from build123d import *

# Parameters (mm, degrees)
F0_R           = 12.7
F1_DEPTH       = 101.6
F3_R           = 10.16
F4_D           = 6.35
F4_START       = 2.7819668
F4_CSINK_D     = 19.05
F4_CSINK_ANGLE = 44.9


with BuildPart() as f1:
    # F0 (on Top) → F1 (new body)
    with BuildSketch(Plane.XY):
        Circle(F0_R)
    extrude(amount=-F1_DEPTH)

    # F3
    f3_edges = [f1.edges().sort_by_distance(p)[0] for p in [
        (-12.7, 0, -101.6),
    ]]
    fillet(f3_edges, radius=F3_R)

    # F4 (through all)
    # its depths count from where the whole tool has entered the part; down to there all is cleared
    with Locations(Plane(origin=(0, 0, -101.6), x_dir=(1, 0, 0), z_dir=(0, 0, -1)).offset(-F4_START)):
        with Locations((0, 0)):
            CounterSinkHole(F4_D / 2, F4_CSINK_D / 2, counter_sink_angle=F4_CSINK_ANGLE)


solid = f1.part
Could you check a few things on this model? Use its own coordinates, in mm. Round coordinates to 2 decimals unless told otherwise and drop trailing zeros. Write each loop counter-clockwise with the first axis right and the second up, starting at its lowest first coordinate (ties: lowest second). Pieces come first, ordered by that corner, then holes. Notation, with made-up numbers: (-21.75, 9.5) - (11.25, 9.5) arc R23 cw to (11.25, 46.5) - close; hole circle Ø2 at (-29.5, 7.5). An arc over 180 degrees is marked (long way). Use a Markdown table: item, result.
Q1. For pin 1 (1 mm diameter, centred on x = 1.5, z = -73.5, fed in from -Y); pin 2 (4 mm diameter, centred on x = -2.5, y = 6, fed in from -Z), each with a flat end and sliding along its axis, tell me the tip position at first contact or that it passes through.
Output values:
| item | result |
|---|---|
| pin 1 | y = -12.66 |
| pin 2 | z = -96.34 |
Q2. Thinking about a two-plate mould opening in X: for faces 1 (the cylindrical face through (-2.75, -12.4, -45.08)), 2 (the cylindrical face through (0.69, 3.1, -41.14)), 3 (the flat face through (3, -3, 0)), which applies, released by +X, released by -X, zero draft, split by the parting line, or undercut?
Output values:
| item | result |
|---|---|
| face 1 | split by the parting line |
| face 2 | undercut |
| face 3 | zero draft |
Q3. I want a section at A-A (z = -44.5). List the corners of the cut face in (x, y) for me (3 decimals), plus the area to 3 significant figures.
Output values:
| item | result |
|---|---|
| outline | circle Ø25.4 at (0, 0); hole circle Ø6.35 at (0, 0) |
| area | 475 mm2 |
Q4. Please list where these lines run through material, in increasing order: L1, parallel to Y at x = 0, z = -17 (3 decimals); L2, parallel to X at y = 1.25, z = -80.5; L3, parallel to Y at x = -2.5, z = -27.5.
Output values:
| item | result |
|---|---|
| L1 | -12.7 to -3.175, 3.175 to 12.7 |
| L2 | -12.64 to -2.92, 2.92 to 12.64 |
| L3 | -12.45 to -1.96, 1.96 to 12.45 |
